```python
from build123d import *

# Parameters (mm, degrees)
EXTRUDE_5_DEPTH     = 50
SHELL_4_T           = -1.75
SKETCH_3_R          = 8
SKETCH_3_R_2        = 1.5
CUT_EXTRUDE_2_DEPTH = 5
SKETCH_5_R          = 1.5
CUT_EXTRUDE_3_DEPTH = 5
SKETCH_6_W          = 5
SKETCH_6_H          = 5
SKETCH_6_R          = 1.5
SKETCH_6_H_2        = 5.539841266
EXTRUDE_8_DEPTH     = 2
SKETCH_9_W          = 9.945628491
SKETCH_9_H          = 14.246438642
CUT_EXTRUDE_4_DEPTH = 15


with BuildPart() as part:
    # 草图1 → 凸台-拉伸5 (new body)
    with BuildSketch(Plane(origin=(0, 0, 0), x_dir=(1, 0, 0), z_dir=(0, 1, 0))):
        with BuildLine():
            Line((0, -52), (26, -52))
            Line((26, -52), (52, -26))
            Line((52, -26), (52, 26))
            Line((52, 26), (26, 52))
            Line((26, 52), (0, 52))
            ThreePointArc((0, 52), (-52, 0), (0, -52))
        make_face()
    extrude(amount=EXTRUDE_5_DEPTH)

    # 抽壳4
    shell_4_openings = [part.faces().sort_by_distance(p)[0] for p in [
        (1.957361837, 50, 0),
    ]]
    offset(amount=SHELL_4_T, openings=shell_4_openings, kind=Kind.INTERSECTION)

    # 草图3 → 切除-拉伸2 (cut)
    with BuildSketch(Plane(origin=(0, 1.75, 0), x_dir=(1, 0, 0), z_dir=(0, 1, 0))):
        with Locations(Location((-32, 0, 0), (0, 0, 270))):
            Circle(SKETCH_3_R)
        with Locations(Location((45, 0, 0), (0, 0, 270))):
            Circle(SKETCH_3_R_2)
        with Locations(Location((-22.5, 38.97114317, 0), (0, 0, 270))):
            Circle(SKETCH_3_R_2)
        with Locations(Location((-22.5, -38.97114317, 0), (0, 0, 270))):
            Circle(SKETCH_3_R_2)
    extrude(amount=-CUT_EXTRUDE_2_DEPTH, mode=Mode.SUBTRACT)

    # 草图5 → 切除-拉伸3 (cut)
    with BuildSketch(Plane(origin=(52, 0, 0), x_dir=(0, 0, -1), z_dir=(1, 0, 0))):
        with Locations((22.5, 25)):
            Circle(SKETCH_5_R)
        with Locations((-22.5, 25)):
            Circle(SKETCH_5_R)
    extrude(amount=-CUT_EXTRUDE_3_DEPTH, mode=Mode.SUBTRACT)

    # 草图6 → 凸台-拉伸8 (add)
    # profile 1 of 4: a face of its own
    with BuildSketch(Plane(origin=(0, 50, 0), x_dir=(1, 0, 0), z_dir=(0, 1, 0))):
        with Locations((54.5, 0)):
            Rectangle(SKETCH_6_W, SKETCH_6_H)
        with Locations(Location((54.5, 0, 0), (0, 0, 270))):
            Circle(SKETCH_6_R, mode=Mode.SUBTRACT)
    # profile 2 of 4: a face of its own
    with BuildSketch(Plane(origin=(0, 50, 0), x_dir=(1, 0, 0), z_dir=(0, 1, 0))):
        with Locations((-54.43986908, 0)):
            Rectangle(SKETCH_6_W, SKETCH_6_H)
        with Locations(Location((-54.5, 0, 0), (0, 0, 270))):
            Circle(SKETCH_6_R, mode=Mode.SUBTRACT)
    # profile 3 of 4: a face of its own
    with BuildSketch(Plane(origin=(0, 50, 0), x_dir=(1, 0, 0), z_dir=(0, 1, 0))):
        Polygon((2.5, 52), (2.5, 57), (-2.5, 57), (-2.5, 52), (-2.5, 51.633473504), (2.5, 51.633473504), align=None)
        with Locations(Location((0, 54.5, 0), (0, 0, 270))):
            Circle(SKETCH_6_R, mode=Mode.SUBTRACT)
    # profile 4 of 4: a face of its own
    with BuildSketch(Plane(origin=(0, 50, 0), x_dir=(1, 0, 0), z_dir=(0, 1, 0))):
        with Locations((0, -54.230079367)):
            Rectangle(SKETCH_6_W, SKETCH_6_H_2)
        with Locations(Location((0, -54.5, 0), (0, 0, 270))):
            Circle(SKETCH_6_R, mode=Mode.SUBTRACT)
    extrude(amount=-EXTRUDE_8_DEPTH)

    # 草图9 → 切除-拉伸4 (cut)
    with BuildSketch(Plane(origin=(-29.751362544, 0, -29.718537282), x_dir=(-0.7067163758191224, 0, 0.707496971123612), z_dir=(-0.707496971123612, 0, -0.7067163758191224))):
        with Locations((0.350985127, 44.684979675)):
            Rectangle(SKETCH_9_W, SKETCH_9_H)
    extrude(amount=CUT_EXTRUDE_4_DEPTH, mode=Mode.SUBTRACT)


solid = part.part
```
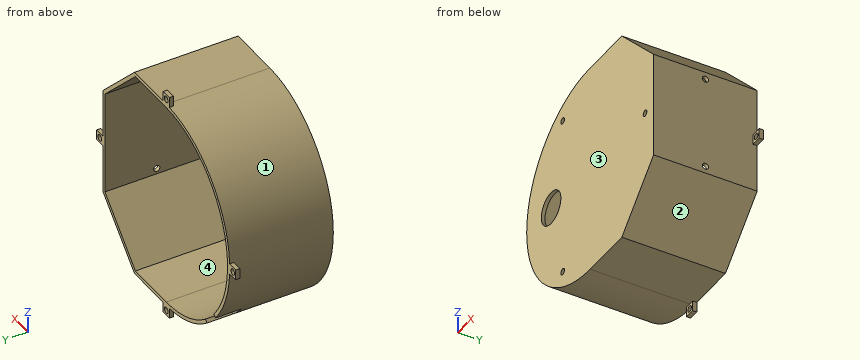
Source: CAD feature listing. Evaluate the final solid. Frame: model axes, mm. Face numbers are marked on the shaded views. Round coordinates to 2 decimals unless told otherwise and drop trailing zeros. Write each loop counter-clockwise with the first axis right and the second up, starting at its lowest first coordinate (ties: lowest second). Pieces come first, ordered by that corner, then holes. Notation, with made-up numbers: M 8,8.5 L 62,8.5 A10 cw 62,24.5 Z; hole C 22.25,9.5 d9. An arc over 180 degrees is marked long. Answer as a JSON object with one key per item and string values. Group by question number.
(1) Section query D-D on x = 20. Output: boundary loops of the cut face in (y, z).
(2) First-contact query: pin 1 (2 mm diameter, centred on x = -44.5, z = 31, fed in from -Y); pin 2 (12.5 mm diameter, centred on x = 13, y = 29, fed in from +Z); pin 3 (5 mm diameter, centred on x = -22.5, z = -38.97, fed in from +Y); pin 4 (4 mm diameter, centred on y = 25, z = 22.5, fed in from -X). Flat tips, straight axial feed; report the tip coordinate or a pass-through.
(3) Section query C-C on y = 25. Output: boundary loops of the cut face in (x, z), then the cut area to 3 significant figures.
(4) Section query A-A on x = -54.5. Output: boundary loops of the cut face in (y, z).
(5) Ray query, line 1 (X direction, y = 48.85, z = 0); line 2 (X direction, y = 48.9, z = 54.5); line 3 (Z direction, x = 6, y = 33.5). Return the intervals inside material, ascending. Write a range as [from, to].
(6) Section query B-B on z = -54.5. Output: boundary loops of the cut face in (x, y), then the cut area to 3 significant figures.
(7) Mould query, pull axis Z, two halves, no side actions, for the marked faces 1, 2, 3 and 4. Classes: +Z half, -Z half, draft (parallel to the pull), parting line (faces both ways), or undercut.
Computed values:
{
 "1": {"outline": "M 0,-52 L 50,-52 L 50,-50.25 L 1.75,-50.25 L 1.75,50.25 L 50,50.25 L 50,52 L 0,52 Z"},
 "2": {"pin 1": "through", "pin 2": "z = 52", "pin 3": "y = 1.75", "pin 4": "x = -47.79"},
 "3": {"outline": "M 0,-52 L 26,-52 L 52,-26 L 52,-24 L 50.25,-24 L 50.25,-25.28 L 25.28,-50.25 L 0,-50.25 A50.25 cw 0,50.25 L 25.28,50.25 L 50.25,25.28 L 50.25,24 L 52,24 L 52,26 L 26,52 L 0,52 A52 ccw Z; M 50.25,-21 L 52,-21 L 52,21 L 50.25,21 Z", "area": "576 mm^2"},
 "4": {"outline": "M 48,-2.5 L 50,-2.5 L 50,-1.5 L 48,-1.5 Z; M 48,1.5 L 50,1.5 L 50,2.5 L 48,2.5 Z"},
 "5": {"line 1": "[-56.94, -56], [-53, -50.25], [50.25, 53], [56, 57]", "line 2": "[-2.5, -1.5], [1.5, 2.5]", "line 3": "[-52, -50.25], [50.25, 52]"},
 "6": {"outline": "M -2.5,48 L -1.5,48 L -1.5,50 L -2.5,50 Z; M 1.5,48 L 2.5,48 L 2.5,50 L 1.5,50 Z", "area": "4.00 mm^2"},
 "7": {"face 1": "parting line", "face 2": "-Z half", "face 3": "draft", "face 4": "undercut"}
}
